Can you work these out from the model? Positions are in its coordinate system, mm. A direction names the side the tool comes from. Give positions to 0.01 mm unless a question says otherwise; leave off trailing zeros. Order: outer loops, then holes, each group sorted by start corner. A loop starts at its lowest first (then second) coordinate and runs counter-clockwise, first axis right, second up. Notation, with made-up numbers: (82, 77.25) - (133, 77.25) arc R10 ccw to (133, 87.25) - close; hole circle Ø6 at (50, 50.25). An arc over 180 degrees is marked (long way). Return JSON: item names as keys, results as strings.
```python
from build123d import *

# Parameters (mm, degrees)
BOSS_EXTRUDE1_DEPTH = 3
FILLET1_R           = 5
FILLET2_R           = 2.5


with BuildPart() as part:
    # Sketch1 → Boss-Extrude1 (new body)
    with BuildSketch(Plane.XY):
        Polygon((-5, -25), (-5, -159), (-25, -159), (-25, -169), (-16.1, -169), (-16.1, -166.5), (-18.6, -166.5), (-18.6, -164.5), (-16.1, -164.5), (-16.1, -162), (-13.9, -162), (-13.9, -164.5), (-11.4, -164.5), (-11.4, -166.5), (-13.9, -166.5), (-13.9, -169), (-5, -169), (-5, -175), (-1.5, -175), (-1.5, -159), (1.5, -159), (1.5, -175), (5, -175), (5, -169), (13.9, -169), (13.9, -166.5), (11.4, -166.5), (11.4, -164.5), (13.9, -164.5), (13.9, -162), (16.1, -162), (16.1, -164.5), (18.6, -164.5), (18.6, -166.5), (16.1, -166.5), (16.1, -169), (25, -169), (25, -159), (5, -159), (5, -25), (20, -25), (20, 25), (0, 25), (-20, 25), (-20, -25), align=None)
    extrude(amount=BOSS_EXTRUDE1_DEPTH)

    # Fillet1
    fillet1_edges = [part.edges().sort_by_distance(p)[0] for p in [
        (5, -25, 1.5),
        (5, -159, 1.5),
        (25, -159, 1.5),
        (-25, -159, 1.5),
        (-5, -25, 1.5),
    ]]
    fillet(fillet1_edges, radius=FILLET1_R)

    # Fillet2
    fillet2_edges = [part.edges().sort_by_distance(p)[0] for p in [
        (-20, -25, 1.5),
        (-20, 25, 1.5),
        (20, 25, 1.5),
        (20, -25, 1.5),
    ]]
    fillet(fillet2_edges, radius=FILLET2_R)


solid = part.part
```
1. If I drill on L1, parallel to Y at x = 14.5, z = 2.35; L2, parallel to Y at x = -11, z = 2.25; L3, parallel to X at y = 16.5, z = 1.7, over which ranges is the centre line in solid material (lowest first)? Write a range as [from, to].
Checks:
{"L1": "[-162, -159], [-25, 25]", "L2": "[-169, -159], [-25, 25]", "L3": "[-20, 20]"}
2. Suppose I cut it at A-A (y = -67). List the corners of the cut face in (x, z) for me, plus the area to 3 significant figures.
Checks:
{"outline": "(-5, 0) - (5, 0) - (5, 3) - (-5, 3) - close", "area": "30.0 mm^2"}
3. Suppose I cut it at B-B (y = 12). List the corners of the cut face in (x, z) for me.
Checks:
{"outline": "(-20, 0) - (20, 0) - (20, 3) - (-20, 3) - close"}
4. For pin 1 Ø1.2 at (y, z) = (-163, 1) entering from -X; pin 2 Ø1.5 at (x, z) = (20, 2.5) entering from +Y; pin 3 Ø10 at (x, y) = (14.5, -153) entering from -Z, each with a flat end and sliding along its axis, tell me the tip position at first contact or that it passes through.
Checks:
{"pin 1": "x = -24.98", "pin 2": "y = 24.29", "pin 3": "through"}
5. On a 3-axis mill with a long thin cutter (end or side, diameter ignored), from which of +Z, -Z, +X, -X, +Y, -Y can I reach the whole of each face in a straight line? I mean faces 1 (the face through (-6, -27, 2)), 2 (the face through (-23, -160, 2)), 3 (the face through (6, -27, 2)). Say none if no direction works.
Checks:
{"face 1": "+Z, -Z, -X", "face 2": "+Z, -Z, -X, +Y", "face 3": "+Z, -Z, +X"}
6. Thinking about a two-plate mould opening in Y: for faces 4 (the face through (7, -158, 2)), 5 (the face through (24, -161, 2)), 6 (the face through (-2, -52, 3)), which applies, +Y half, -Y half, draft (parallel to the pull), parting line (faces both ways), or undercut?
Checks:
{"face 4": "undercut", "face 5": "+Y half", "face 6": "draft"}
